from build123d import *

# Parameters (mm, degrees)
SKETCH1_W           = 63.5
SKETCH1_H           = 63.5
SKETCH1_W_2         = 57.15
SKETCH1_H_2         = 57.15
BOSS_EXTRUDE1_DEPTH = 355.6
SKETCH2_R           = 12.7
CUT_EXTRUDE1_DEPTH  = 363.617804996


with BuildPart() as part:
    # Sketch1 → Boss-Extrude1 (new, symmetric)
    with BuildSketch(Plane.XY):
        Rectangle(SKETCH1_W, SKETCH1_H)
        Rectangle(SKETCH1_W_2, SKETCH1_H_2, mode=Mode.SUBTRACT)
    extrude(amount=BOSS_EXTRUDE1_DEPTH, both=True)

    # Sketch2 → Cut-Extrude1 (cut, through all)
    with BuildSketch(Plane.ZY.offset(31.75)):
        with Locations((-323.85, 0)):
            Circle(SKETCH2_R)
    extrude(amount=-CUT_EXTRUDE1_DEPTH, mode=Mode.SUBTRACT)


solid = part.part
The model under review builds one solid part; all positions refer to its coordinate system, in mm. A direction names the side the tool comes from. Round coordinates to 2 decimals unless told otherwise and drop trailing zeros. Loops run counter-clockwise (first coordinate to the right, second up) from the corner with the lowest first, then second, coordinate; pieces in that order, holes last. Notation, with made-up numbers: M 41.5,23 L 73.5,23 A26 cw 73.5,48 Z; hole C 19,12.5 d8. An arc over 180 degrees is marked long. Answer as a JSON object with one key per item and string values.
Item 1: We need section D-D, the plane z = 3. State the section outline as (x, y) points (3 decimals), and give its area (3 significant figures).
Check sheet entries:
{"outline": "M -31.75,-31.75 L 31.75,-31.75 L 31.75,31.75 L -31.75,31.75 Z; hole M -28.575,-28.575 L 28.575,-28.575 L 28.575,28.575 L -28.575,28.575 Z", "area": "766 mm2"}
Item 2: Clearance check with flat-ended pins moving along their axes: P1, Ø15, axis at y = 0, z = -323.85, coming from the -X side; P2, Ø8, axis at x = -25, y = -5, coming from the -Z side. State where each tip first meets the part, or that it passes through.
Check sheet entries:
{"P1": "through", "P2": "z = -355.6"}
Item 3: Tool access review of faces 1 (the face through (-3, -30, -355.6)), 2 (the face through (0, -28.575, 5)): name each direction out of +Z, -Z, +X, -X, +Y, -Y from which nothing blocks a thin tool from reaching the whole face with its end or side.
Check sheet entries:
{"face 1": "-Z, +X, -X, +Y, -Y", "face 2": "+Z, -Z"}
Item 4: For line 1 along Y through (x, z) = (-17.5, -222.5) (3 decimals); line 2 along Y through (x, z) = (-31, -323), list the stretches that pass through material, from the lowest coordinate up.
Check sheet entries:
{"line 1": "-31.75 to -28.575, 28.575 to 31.75", "line 2": "-31.75 to -12.67, 12.67 to 31.75"}
Item 5: We need section A-A, the plane z = -323.85. State the section outline as (x, y) points (3 decimals), and give its area (3 significant figures).
Check sheet entries:
{"outline": "M -31.75,-31.75 L 31.75,-31.75 L 31.75,-12.7 L 28.575,-12.7 L 28.575,-28.575 L -28.575,-28.575 L -28.575,-12.7 L -31.75,-12.7 Z; M -31.75,12.7 L -28.575,12.7 L -28.575,28.575 L 28.575,28.575 L 28.575,12.7 L 31.75,12.7 L 31.75,31.75 L -31.75,31.75 Z", "area": "605 mm2"}
Item 6: We need section B-B, the plane y = 0. State the section outline as (x, z) points (3 decimals), and give its area (3 significant figures).
Check sheet entries:
{"outline": "M -31.75,-355.6 L -28.575,-355.6 L -28.575,-336.55 L -31.75,-336.55 Z; M -31.75,-311.15 L -28.575,-311.15 L -28.575,355.6 L -31.75,355.6 Z; M 28.575,-355.6 L 31.75,-355.6 L 31.75,-336.55 L 28.575,-336.55 Z; M 28.575,-311.15 L 31.75,-311.15 L 31.75,355.6 L 28.575,355.6 Z", "area": "4,350 mm2"}
Item 7: The part is to be moulded in two halves that separate along Y. For faces 3 (the face through (31.75, 0, 5)), 4 (the face through (0, 31.75, 5)), 5 (the face through (-28.575, 0, 5)), say which applies: +Y half, -Y half, draft (parallel to the pull), parting line (faces both ways), or undercut.
Check sheet entries:
{"face 3": "draft", "face 4": "+Y half", "face 5": "undercut"}
Item 8: We need section C-C, the plane x = -17.5. State the section outline as (y, z) points (3 decimals), and give its area (3 significant figures).
Check sheet entries:
{"outline": "M -31.75,-355.6 L -28.575,-355.6 L -28.575,355.6 L -31.75,355.6 Z; M 28.575,-355.6 L 31.75,-355.6 L 31.75,355.6 L 28.575,355.6 Z", "area": "4,520 mm2"}
